Build history of the part. All positions in model axes, mm. A direction names the side the tool comes from. Give positions to 0.01 mm unless a question says otherwise; leave off trailing zeros. Order: outer loops, then holes, each group sorted by start corner. A loop starts at its lowest first (then second) coordinate and runs counter-clockwise, first axis right, second up. Notation, with made-up numbers: M 1,-21 L 19,-21 A32 ccw 19,18 Z; hole C 16.5,7 d1. An arc over 180 degrees is marked long. One line per item, written item: value.
Autodesk Inventor part; units mm, degrees
ref_plane "Work Plane1" through (0, -2.75, 0) normal (0, -1, 0) x (1, 0, 0)
ref_plane "Work Plane2" through (-152.5, -8.5, -20) normal (0, 0, -1) x (-1, 0, 0)
ref_plane "Work Plane3" through (-195, -9.5, -21.5) normal (0, 0, -1) x (-1, 0, 0)
sketch "Sketch1" plane through (0, 0, 0) normal (0, 1, 0) x (-1, 0, 0)
  line L0 (0, 0) -> (220, 0)
  line L1 (220, 0) -> (220, -43)
  line L2 (220, -43) -> (0, -43)
  line L3 (0, -43) -> (0, 0)
  line L4 (10, -12.5) -> (30, -12.5)
  line L5 (30, -12.5) -> (30, -32.5)
  line L6 (30, -32.5) -> (10, -32.5)
  line L7 (10, -32.5) -> (10, -12.5)
  circle A0 centre (10, -12.5) radius 1.5
  circle A1 centre (30, -32.5) radius 1.5
  circle A2 centre (30, -12.5) radius 1.5
  circle A3 centre (10, -32.5) radius 1.5
  line L8 (220, 0) -> (195, 0)
  line L9 (195, 0) -> (195, -43)
  line L10 (195, -43) -> (220, -43)
  line L11 (220, -43) -> (220, 0)
  line L12 (195, -4) -> (0, -4)
  line L13 (0, -4) -> (0, -39)
  line L14 (0, -39) -> (195, -39)
  line L15 (195, -39) -> (195, -4)
  line L16 (36, -4) -> (36, -39)
  point P0 (195, 0)
  point P1 (0, -4)
  dimension "d0" = 220
  dimension "d1" = 43
  dimension "d2" = 20
  dimension "d3" = 20
  dimension "d4" = 12.5
  dimension "d5" = 10
  dimension "d6" = 3
  dimension "d7" = 3
  dimension "d8" = 3
  dimension "d9" = 3
  dimension "d18" = 4
  dimension "d19" = 4
  dimension "d23" = 36
  dimension "d66" = 25
extrude "Extrusion1" add sketch "Sketch1" along normal blind 4 contours L0 L1 L2 L9 | L12 L16 L14 L3 | L9 L14 L16 L12 | L4 A2 L5 A1 L6 A3 L7 A0
extrude "Extrusion2" add sketch "Sketch1" against normal blind 5.5 contours L0 L1 L2 L9 | L9 L14 L16 L12
ref_plane "Work Plane1" through (0, -2.75, 0) normal (0, -1, 0) x (1, 0, 0)
mirror "Mirror1" about plane through (0, -2.75, 0) normal (0, -1, 0) of "Extrusion1"
chamfer "Chamfer1" distance 7.5 angle 45 4 edges at (0, 2, -4) (0, -7.5, -4) (0, -7.5, -39) (0, 2, -39)
ref_plane "Work Plane2" through (-152.5, -8.5, -20) normal (0, 0, -1) x (-1, 0, 0)
sketch "Sketch5" plane through (-195, -9.5, -39) normal (0, -1, 0) x (1, 0, 0)
  circle A0 centre (165, 26.5) radius 1.5
  line L0 (165, 29.9641) -> (168, 28.2321)
  line L1 (168, 28.2321) -> (168, 24.7679)
  line L2 (168, 24.7679) -> (165, 23.0359)
  line L3 (165, 23.0359) -> (162, 24.7679)
  line L4 (162, 24.7679) -> (162, 28.2321)
  line L5 (162, 28.2321) -> (165, 29.9641)
  circle A1 centre (185, 26.5) radius 1.5
  line L6 (185, 29.9641) -> (188, 28.2321)
  line L7 (188, 28.2321) -> (188, 24.7679)
  line L8 (188, 24.7679) -> (185, 23.0359)
  line L9 (185, 23.0359) -> (182, 24.7679)
  line L10 (182, 24.7679) -> (182, 28.2321)
  line L11 (182, 28.2321) -> (185, 29.9641)
  circle A2 centre (185, 6.5) radius 1.5
  line L12 (185, 9.9641) -> (188, 8.2321)
  line L13 (188, 8.2321) -> (188, 4.7679)
  line L14 (188, 4.7679) -> (185, 3.0359)
  line L15 (185, 3.0359) -> (182, 4.7679)
  line L16 (182, 4.7679) -> (182, 8.2321)
  line L17 (182, 8.2321) -> (185, 9.9641)
  circle A3 centre (165, 6.5) radius 1.5
  line L18 (165, 9.9641) -> (168, 8.2321)
  line L19 (168, 8.2321) -> (168, 4.7679)
  line L20 (168, 4.7679) -> (165, 3.0359)
  line L21 (165, 3.0359) -> (162, 4.7679)
  line L22 (162, 4.7679) -> (162, 8.2321)
  line L23 (162, 8.2321) -> (165, 9.9641)
  circle A4 centre (165, 26.5) radius 5.25
  circle A5 centre (185, 26.5) radius 5.25
  circle A6 centre (185, 6.5) radius 5.25
  circle A7 centre (165, 6.5) radius 5.25
  point P0 (195, 39)
  dimension "d44" = 6
  dimension "d45" = 6
  dimension "d46" = 6
  dimension "d47" = 6
  dimension "d48" = 10.5
  dimension "d49" = 10.5
  dimension "d50" = 10.5
  dimension "d51" = 10.5
extrude "Extrusion5" add sketch "Sketch5" along normal blind 3.5 contours A4 | A5 | A6 | A7
sketch "Sketch6" plane through (-195, -9.5, -39) normal (0, -1, 0) x (1, 0, 0)
  circle A0 centre (65, 7.5) radius 1.5
  line L0 (187.5, 0) -> (0, 0)
  line L1 (0, 0) -> (0, -4)
  circle A1 centre (85, 7.5) radius 1.5
  circle A2 centre (105, 7.5) radius 1.5
  circle A3 centre (125, 7.5) radius 1.5
  point P0 (195, 39)
  point P1 (0, -5)
  dimension "d54" = 3
  dimension "d55" = 7.5
  dimension "d56" = 65
  dimension "d59" = 20
extrude "Extrusion6" cut sketch "Sketch6" against normal blind 33.25
ref_plane "Work Plane3" through (-195, -9.5, -21.5) normal (0, 0, -1) x (-1, 0, 0)
mirror "Mirror2" about plane through (-195, -9.5, -21.5) normal (0, 0, -1) of "Extrusion6"
sketch "Sketch7" plane through (-220, 4, 0) normal (0, 0, 1) x (1, 0, 0)
  point P0 (220, -4)
ref_plane "Work Plane4" through (-195, -9.5, -21.5) normal (0, 0, 1) x (1, 0, 0)
sketch "Sketch9" plane through (-220, 4, 0) normal (0, 0, 1) x (1, 0, 0)
  circle A0 centre (7.5, -6.75) radius 2
  line L0 (0, -13.5) -> (0, 0)
  line L1 (0, 0) -> (25, 0)
  point P0 (220, -4)
  dimension "d75" = 4
  dimension "d76" = 7.5
  dimension "d77" = 6.75
extrude "Extrusion8" cut sketch "Sketch9" against normal blind 73.25
sketch "Sketch10" plane through (0, 4, 0) normal (0, 1, 0) x (1, 0, 0)
  circle A0 centre (-195, 31.5) radius 1.5
  circle A1 centre (-195, 11.5) radius 1.5
  circle A2 centre (-90, 11.5) radius 1.5
  circle A3 centre (-110, 11.5) radius 1.5
  circle A4 centre (-70, 11.5) radius 1.5
  circle A5 centre (-130, 11.5) radius 1.5
  circle A6 centre (-90, 31.5) radius 1.5
  circle A7 centre (-110, 31.5) radius 1.5
  circle A8 centre (-70, 31.5) radius 1.5
  circle A9 centre (-130, 31.5) radius 1.5
  line L0 (-7.5, 39) -> (0, 31.5)
  line L1 (-7.5, 39) -> (-195, 39)
  line L2 (-195, 39) -> (-195, 43)
  line L3 (-195, 43) -> (-220, 43)
  line L4 (-220, 43) -> (-220, 0)
  line L5 (-220, 0) -> (-195, 0)
  line L6 (-195, 0) -> (-195, 4)
  line L7 (-195, 4) -> (-7.5, 4)
  line L8 (0, 11.5) -> (-7.5, 4)
  line L9 (0, 11.5) -> (0, 31.5)
  circle A10 centre (-10, 32.5) radius 1.5
  circle A11 centre (-30, 32.5) radius 1.5
  circle A12 centre (-30, 12.5) radius 1.5
  circle A13 centre (-10, 12.5) radius 1.5
  point P0 (0, 0)
  dimension "d80" = 65
  dimension "d81" = 3
  dimension "d82" = 3
extrude "Extrusion9" cut sketch "Sketch10" against normal blind 23.75 contours A0 | A1
properties part number "RobotBaseMotorExt"
1) Pin check, flat tips, straight feed: pin 1 (1.8 mm diameter, centred on x = -110, z = -11.5, fed in from -Y); pin 2 (5 mm diameter, centred on x = -195, z = -11.5, fed in from -Y); pin 3 (2 mm diameter, centred on y = -2, z = -22, fed in from +X); pin 4 (1.7 mm diameter, centred on y = -12, z = -33, fed in from +X). Stop position of each tip, or through.
Check values:
pin 1: through
pin 2: y = -9.5
pin 3: x = -36
pin 4: x = -4.75
2) Saw through at B-B, the plane z = -22.5. Write the cut outline in (x, y), then the cut area to 3 significant figures.
Check values:
outline: M -220,-9.5 L 0,-9.5 L 0,-5.5 L -36,-5.5 L -36,0 L 0,0 L 0,4 L -220,4 Z; hole C -212.5,-2.75 d4
area: 2,760 mm^2
3) Saw through at C-C, the plane x = -171. Write the cut outline in (y, z), then the cut area to 4 significant figures.
Check values:
outline: M -9.5,-39 L 4,-39 L 4,-4 L -9.5,-4 Z
area: 472.5 mm^2
4) Tool access for faces 1 (the face through (-208, -3, -43)), 2 (the face through (-33, -11, -13)), 3 (the face through (-195, -3, -41)), 4 (the face through (-195, -3, -2)): list every direction of +Z, -Z, +X, -X, +Y, -Y with a clear straight run to the whole face (end or side of a thin tool).
Check values:
face 1: -Z, +X, -X, +Y, -Y
face 2: -Y
face 3: -Z, +X, +Y, -Y
face 4: +Z, +X, +Y, -Y
5) Drill centre lines: probe 1 along Z at (x, y) = (-90, -3); probe 2 along Y at (x, z) = (-16.5, -17.5); probe 3 along X at (y, z) = (-10.5, -34). Where is each one in solid material? Low to high. Write a range as from..to.
Check values:
probe 1: -39..-33, -30..-13, -10..-4
probe 2: -9.5..-5.5, 0..4
probe 3: -35.03..-33, -27..-24.97, -15.03..-13, -7..-4.97
6) Saw through at A-A, the plane x = -212.5. Write the cut outline in (y, z), then the cut area to 4 significant figures.
Check values:
outline: M -9.5,-43 L -4.75,-43 L -4.75,0 L -9.5,0 Z; M -0.75,-43 L 4,-43 L 4,0 L -0.75,0 Z
area: 408.5 mm^2
7) Mould opens along X. For faces 5 (the face through (-220, -3, -21)), 6 (the face through (-108, 4, -21)), 7 (the face through (-214.5, -2.7, -21.2)) say: released by +X, released by -X, zero draft, split by the parting line, or undercut.
Check values:
face 5: released by -X
face 6: zero draft
face 7: undercut
